```python
from build123d import *

# Parameters (mm, degrees)
BOSS_EXTRUDE1_DEPTH = 50
SKETCH2_W           = 50
SKETCH2_H           = 8
CUT_EXTRUDE1_DEPTH  = 2
SKETCH4_W           = 45
SKETCH4_H           = 52
CUT_EXTRUDE2_DEPTH  = 16
SKETCH6_R           = 1.5
CUT_EXTRUDE4_DEPTH  = 2
CUT_EXTRUDE_2_DEPTH = 16


with BuildPart() as part:
    # Sketch1 → Boss-Extrude1 (new body)
    with BuildSketch(Plane.XY):
        Polygon((-10, 0), (10, 0), (10, 55), (6, 55), (-10, 3), align=None)
    extrude(amount=BOSS_EXTRUDE1_DEPTH)

    # Sketch2 → Cut-Extrude1 (cut)
    with BuildSketch(Plane(origin=(10, 0, 0), x_dir=(0, 0, -1), z_dir=(1, 0, 0))):
        with Locations((-25, 10)):
            Rectangle(SKETCH2_W, SKETCH2_H)
        with Locations((-25, 26)):
            Rectangle(SKETCH2_W, SKETCH2_H)
    extrude(amount=-CUT_EXTRUDE1_DEPTH, mode=Mode.SUBTRACT)

    # Sketch4 → Cut-Extrude2 (cut)
    with BuildSketch(Plane.ZY.offset(10)):
        with Locations((25, 29)):
            Rectangle(SKETCH4_W, SKETCH4_H)
    extrude(amount=-CUT_EXTRUDE2_DEPTH, mode=Mode.SUBTRACT)

    # Sketch6 → Cut-Extrude4 (cut)
    with BuildSketch(Plane(origin=(8, 0, 0), x_dir=(0, 0, -1), z_dir=(1, 0, 0))):
        with Locations((-25, 26)):
            Circle(SKETCH6_R)
        with Locations((-25, 10)):
            Circle(SKETCH6_R)
    extrude(amount=-CUT_EXTRUDE4_DEPTH, mode=Mode.SUBTRACT)

    # 草图2 → 切除-拉伸2 (cut)
    with BuildSketch(Plane(origin=(0, 3, 0), x_dir=(1, 0, 0), z_dir=(0, 1, 0))):
        with BuildLine():
            Line((-7, -24), (3, -24))
            ThreePointArc((3, -24), (4, -25), (3, -26))
            Line((3, -26), (-7, -26))
            ThreePointArc((-7, -26), (-8, -25), (-7, -24))
        make_face()
    extrude(amount=-CUT_EXTRUDE_2_DEPTH, mode=Mode.SUBTRACT)


solid = part.part
```
Input: part model. Units: mm. Frame: model coordinates. A direction names the side the tool comes from. Round coordinates to 2 decimals unless told otherwise and drop trailing zeros. Loops run counter-clockwise (first coordinate to the right, second up) from the corner with the lowest first, then second, coordinate; pieces in that order, holes last. Notation, with made-up numbers: (-18.5, 17.5) -> (6.5, 17.5) arc R26 ccw to (6.5, 45.5) -> close; hole circle Ø4 at (-27, 0.5). An arc over 180 degrees is marked (long way). One line per item, written item: value.
(1) Section D-D (z = 39.5). Return the cut outline in (x, y).
Geometry check:
outline: (-10, 0) -> (10, 0) -> (10, 6) -> (8, 6) -> (8, 14) -> (10, 14) -> (10, 22) -> (8, 22) -> (8, 30) -> (10, 30) -> (10, 55) -> (6, 55) -> (6, 3) -> (-10, 3) -> close
(2) Section C-C (y = 10). Return the cut outline in (x, z), plus the area to 3 significant figures.
Geometry check:
outline: (-7.85, 0) -> (8, 0) -> (8, 23.5) -> (6, 23.5) -> (6, 2.5) -> (-7.85, 2.5) -> close; (-7.85, 47.5) -> (6, 47.5) -> (6, 26.5) -> (8, 26.5) -> (8, 50) -> (-7.85, 50) -> close
area: 163 mm2
(3) Set-up query: faces 1 (the face through (1, 17, 2.5)), 2 (the face through (-8, 2, 25)), 3 (the face through (10, 18, 25)), 4 (the face through (8, 12, 25)). Return all of +Z, -Z, +X, -X, +Y, -Y with unobstructed straight access to the full face (end or side cutting, diameter ignored); none if empty.
Geometry check:
face 1: -X, +Y
face 2: +Y, -Y
face 3: +Z, -Z, +X, +Y, -Y
face 4: +Z, -Z, +X
(4) Mould query, pull axis X, two halves, no side actions, for faces 5 (the face through (-2, 2, 24)), 6 (the face through (7.01, 10.07, 26.5)), 7 (the face through (6, 29, 25)). Classes: pulls with the +X half, pulls with the -X half, needs draft (parallel to the pull), parting line crosses it, or undercut.
Geometry check:
face 5: undercut
face 6: needs draft
face 7: pulls with the -X half
(5) Material intervals for line 1 (Y direction, x = 6.65, z = 25); line 2 (Z direction, x = 0.5, y = 12.5); line 3 (Y direction, x = -9, z = 30), sorted ascending. Write a range as [from, to].
Geometry check:
line 1: [0, 8.5], [11.5, 24.5], [27.5, 55]
line 2: [0, 2.5], [47.5, 50]
line 3: [0, 3]
(6) Section B-B (x = 1). Return the cut outline in (y, z), plus the area to 3 significant figures.
Geometry check:
outline: (0, 0) -> (38.75, 0) -> (38.75, 2.5) -> (3, 2.5) -> (3, 24) -> (0, 24) -> close; (0, 26) -> (3, 26) -> (3, 47.5) -> (38.75, 47.5) -> (38.75, 50) -> (0, 50) -> close
area: 323 mm2
(7) Pin query (flat end, axial travel): pin 1 (1 mm diameter, centred on y = 48.5, z = 27, fed in from -X); pin 2 (8 mm diameter, centred on x = 1.5, z = 28, fed in from +Y); pin 3 (4 mm diameter, centred on y = 26.5, z = 30.5, fed in from +X). Return the tip coordinate at first contact, or that it passes through.
Geometry check:
pin 1: x = 6
pin 2: y = 3
pin 3: x = 8
(8) Section A-A (z = 25). Return the cut outline in (x, y), plus the area to 3 significant figures.
Geometry check:
outline: (-10, 0) -> (-8, 0) -> (-8, 3) -> (-10, 3) -> close; (4, 0) -> (10, 0) -> (10, 6) -> (8, 6) -> (8, 8.5) -> (6, 8.5) -> (6, 3) -> (4, 3) -> close; (6, 11.5) -> (8, 11.5) -> (8, 14) -> (10, 14) -> (10, 22) -> (8, 22) -> (8, 24.5) -> (6, 24.5) -> close; (6, 27.5) -> (8, 27.5) -> (8, 30) -> (10, 30) -> (10, 55) -> (6, 55) -> close
area: 188 mm2
